from build123d import *

# Parameters (mm, degrees)
PAD_DEPTH       = 8
SKETCH001_R     = 26
POCKET_DEPTH    = 8.001
POCKET001_DEPTH = 8.001
POCKET002_DEPTH = 8.001
POCKET003_DEPTH = 8.001
POCKET004_DEPTH = 8.001
SKETCH006_R     = 26
SKETCH006_R_2   = 24.5
PAD001_DEPTH    = 2


with BuildPart() as part:
    # Sketch → Pad (new body)
    with BuildSketch(Plane.XY):
        with BuildLine():
            Line((-41, 39), (-41, -26))
            ThreePointArc((-41, -26), (-36.606602, -36.606602), (-26, -41))
            Line((-26, -41), (39, -41))
            ThreePointArc((39, -41), (40.414214, -40.414214), (41, -39))
            Line((41, -39), (41, 39))
            ThreePointArc((41, 39), (40.414214, 40.414214), (39, 41))
            Line((39, 41), (-39, 41))
            ThreePointArc((-39, 41), (-40.414214, 40.414214), (-41, 39))
        make_face()
    extrude(amount=PAD_DEPTH)

    # Sketch001 (on DatumPlane) → Pocket (cut, through all)
    with BuildSketch(Plane.XY.offset(8)):
        with Locations((-1, -1)):
            Circle(SKETCH001_R)
    extrude(amount=-POCKET_DEPTH, mode=Mode.SUBTRACT)

    # Sketch002 (on DatumPlane) → Pocket001 (cut, through all)
    with BuildSketch(Plane.XY.offset(8)):
        with BuildLine():
            Line((-26, -36), (32.125, -36))
            Line((32.125, -36), (19.651021, -24.12002))
            ThreePointArc((-21.081146, -24.61668), (-0.622036, -31.997696), (19.651021, -24.12002))
            Line((-21.081146, -24.61668), (-31.078765, -34.614299))
            ThreePointArc((-31.078765, -34.614299), (-28.632205, -35.647357), (-26, -36))
        make_face()
    extrude(amount=-POCKET001_DEPTH, mode=Mode.SUBTRACT)

    # Sketch003 (on DatumPlane) → Pocket002 (cut, through all)
    with BuildSketch(Plane.XY.offset(8)):
        with BuildLine():
            ThreePointArc((-36, -26), (-35.647357, -28.632205), (-34.614299, -31.078765))
            Line((-34.614299, -31.078765), (-24.61668, -21.081146))
            ThreePointArc((-24.12002, 19.651021), (-31.997696, -0.622036), (-24.61668, -21.081146))
            Line((-36, 32.125), (-24.12002, 19.651021))
            Line((-36, 32.125), (-36, -26))
        make_face()
    extrude(amount=-POCKET002_DEPTH, mode=Mode.SUBTRACT)

    # Sketch004 (on DatumPlane) → Pocket003 (cut, through all)
    with BuildSketch(Plane.XY.offset(8)):
        with BuildLine():
            Line((-32.785714, 36), (32.464466, 36))
            Line((32.464466, 36), (19.081146, 22.61668))
            ThreePointArc((19.081146, 22.61668), (-0.622036, 29.997696), (-20.49933, 23.099297))
            Line((-20.49933, 23.099297), (-32.785714, 36))
        make_face()
    extrude(amount=-POCKET003_DEPTH, mode=Mode.SUBTRACT)

    # Sketch005 (on DatumPlane) → Pocket004 (cut, through all)
    with BuildSketch(Plane.XY.offset(8)):
        with BuildLine():
            Line((36, 32.464466), (36, -32.785714))
            Line((36, -32.785714), (23.099297, -20.49933))
            ThreePointArc((23.099297, -20.49933), (29.997696, -0.622036), (22.61668, 19.081146))
            Line((36, 32.464466), (22.61668, 19.081146))
        make_face()
    extrude(amount=-POCKET004_DEPTH, mode=Mode.SUBTRACT)

    # Sketch006 → Pad001 (join)
    with BuildSketch(Plane.XY):
        with Locations((-1, -1)):
            Circle(SKETCH006_R)
        with Locations((-1, -1)):
            Circle(SKETCH006_R_2, mode=Mode.SUBTRACT)
    extrude(amount=PAD001_DEPTH)


solid = part.part
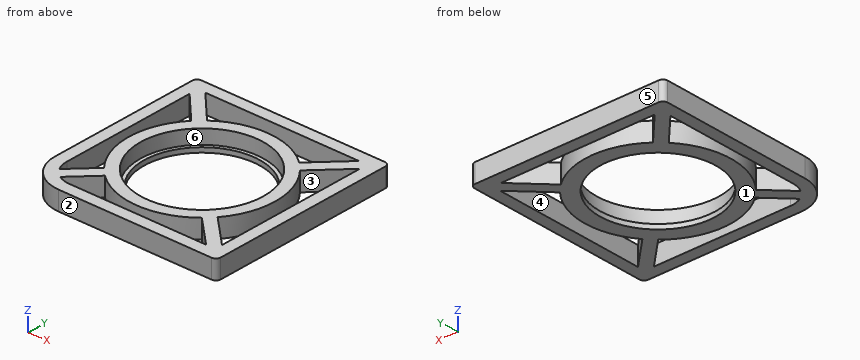
Input: part model. Units: mm. Frame: model coordinates. Face numbers are marked on the shaded views. A direction names the side the tool comes from. Round coordinates to 2 decimals unless told otherwise and drop trailing zeros. Write each loop counter-clockwise with the first axis right and the second up, starting at its lowest first coordinate (ties: lowest second). Pieces come first, ordered by that corner, then holes.
1) Cut plane A-A (z = 3.25). Return the cut outline in (x, y) (3 decimals), then the cut area to 3 significant figures.
2) Draft query along Y for the marked faces 1, 2 and 3. Return one class per face: pulls with the +Y half, pulls with the -Y half, needs draft (parallel to the pull), parting line crosses it, or undercut.
3) Cut plane D-D (x = 35). Return the cut outline in (y, z), then the cut area to 3 significant figures.
4) Cut plane B-B (x = -1). Return the cut outline in (y, z).
5) Ray query, L1, parallel to Y at x = -1, z = 1.55; L2, parallel to Y at x = -1, z = 5.6; L3, parallel to X at y = -17, z = 6.5. Return the intervals inside material, ascending.
6) Reachability of the marked faces 4, 5 and 6 from +Z, -Z, +X, -X, +Y, -Y: full face, straight path, thin tool, end or side. Return the list, or none.
Geometry says:
1. outline: (-41, -26) arc R15 ccw to (-26, -41) - (39, -41) arc R2 ccw to (41, -39) - (41, 39) arc R2 ccw to (39, 41) - (-39, 41) arc R2 ccw to (-41, 39) - close; hole (-36, -26) arc R10 ccw to (-34.614, -31.079) - (-24.617, -21.081) arc R31 cw to (-24.12, 19.651) - (-36, 32.125) - close; hole (-32.786, 36) - (-20.499, 23.099) arc R31 cw to (19.081, 22.617) - (32.464, 36) - close; hole (-31.079, -34.614) arc R10 ccw to (-26, -36) - (32.125, -36) - (19.651, -24.12) arc R31 cw to (-21.081, -24.617) - close; hole circle Ø52 at (-1, -1); hole (22.617, 19.081) arc R31 cw to (23.099, -20.499) - (36, -32.786) - (36, 32.464) - close
1. area: 2,760 mm2
2. face 1: needs draft
2. face 2: pulls with the -Y half
2. face 3: undercut
3. outline: (-41, 0) - (-31.83, 0) - (-31.83, 8) - (-41, 8) - close; (31.46, 0) - (41, 0) - (41, 8) - (31.46, 8) - close
3. area: 150 mm2
4. outline: (-41, 0) - (-36, 0) - (-36, 8) - (-41, 8) - close; (-32, 0) - (-25.5, 0) - (-25.5, 2) - (-27, 2) - (-27, 8) - (-32, 8) - close; (23.5, 0) - (30, 0) - (30, 8) - (25, 8) - (25, 2) - (23.5, 2) - close; (36, 0) - (41, 0) - (41, 8) - (36, 8) - close
5. L1: y = -41 to -36, -32 to -25.5, 23.5 to 30, 36 to 41
5. L2: y = -41 to -36, -32 to -27, 25 to 30, 36 to 41
5. L3: x = -41 to -36, -27.55 to -21.49, 19.49 to 25.55, 36 to 41
6. face 4: +Z, -Z
6. face 5: +Z, -Z, +X, -X, +Y
6. face 6: +Z
